Check sheet for the modelled part. Datum: model origin and axes. Units: mm. A direction names the side the tool comes from. Coordinates: 2 decimals unless noted, no trailing zeros. Write each loop counter-clockwise with the first axis right and the second up, starting at its lowest first coordinate (ties: lowest second). Pieces come first, ordered by that corner, then holes. Notation, with made-up numbers: (32, -38.5) - (42, -38.5) arc R30 cw to (42, -16.5) - close; hole circle Ø4 at (67, 66.25). An arc over 180 degrees is marked (long way). Write each question's results on one line, items separated by ' | '.
from build123d import *

# Parameters (mm, degrees)
F0_W     = 30.48
F0_H     = 25.4
F0_W_2   = 25.4
F0_H_2   = 20.32
F1_DEPTH = 44.45
F2_W     = 25.4
F2_H     = 20.32
F2_W_2   = 20.32
F2_H_2   = 15.24
F2_R     = 2.159
F3_DEPTH = 25.4
F4_R     = 2.159
F5_DEPTH = 5.08
F6_R     = 3.429
F6_W     = 8.128
F6_H     = 3.048
F7_DEPTH = 25.4
F8_W     = 54.200325
F8_H     = 68.948708
F9_DEPTH = 12.7


with BuildPart() as f1:
    # F0 (on Top) → F1 (new body, symmetric)
    with BuildSketch(Plane.XY):
        Rectangle(F0_W, F0_H)
        Rectangle(F0_W_2, F0_H_2, mode=Mode.SUBTRACT)
    extrude(amount=F1_DEPTH, both=True)

    # F2 (on face) → F3 (join)
    with BuildSketch(Plane.XY.offset(44.45)):
        Rectangle(F2_W, F2_H)
        Rectangle(F2_W_2, F2_H_2, mode=Mode.SUBTRACT)
        Rectangle(F2_W_2, F2_H_2)
        with Locations((-6.35, 0)):
            Circle(F2_R, mode=Mode.SUBTRACT)
        with Locations((6.35, 0)):
            Circle(F2_R, mode=Mode.SUBTRACT)
    extrude(amount=-F3_DEPTH)

    # F4 (on face) → F5 (cut)
    with BuildSketch(Plane(origin=(0, 0, 19.05), x_dir=(1, 0, 0), z_dir=(0, 0, -1))):
        with Locations((6.35, 0)):
            Circle(F4_R)
        with Locations((-6.35, 0)):
            Circle(F4_R)
    extrude(amount=-F5_DEPTH, mode=Mode.SUBTRACT)

    # F6 (on face) → F7 (cut)
    with BuildSketch(Plane.XZ.offset(12.7)):
        with Locations((0, 8.001)):
            Circle(F6_R)
        with Locations((0, -8.4074)):
            Rectangle(F6_W, F6_H)
        with BuildLine():
            Line((-3.2258, -29.3624), (-3.2258, -32.1564))
            Line((-3.2258, -32.1564), (3.2258, -32.1564))
            Line((3.2258, -32.1564), (3.2258, -29.3624))
            ThreePointArc((3.2258, -29.3624), (0, -26.1366), (-3.2258, -29.3624))
        make_face()
    extrude(amount=-F7_DEPTH, mode=Mode.SUBTRACT)

    # F8 (on Front) → F9 (cut, symmetric)
    with BuildSketch(Plane.XZ):
        with Locations((2.120081, 16.499758)):
            Rectangle(F8_W, F8_H)
    extrude(amount=F9_DEPTH, both=True, mode=Mode.SUBTRACT)


solid = f1.part
1. Sectioned sample at D-D (z = -19.5). Record the cut outline in (x, y).
Values follow:
outline: (-15.24, -12.7) - (15.24, -12.7) - (15.24, 12.7) - (-15.24, 12.7) - close; hole (-12.7, -10.16) - (12.7, -10.16) - (12.7, 10.16) - (-12.7, 10.16) - close
2. Material ranges on L1, parallel to X at y = -8.5, z = -26.75; L2, parallel to Y at x = -3, z = -27.5; L3, parallel to X at y = 11, z = -30.5, recorded low to high. Write a range as [from, to].
Values follow:
L1: x = [-15.24, -12.7], [12.7, 15.24] | L2: y = [-12.7, -10.16], [10.16, 12.7] | L3: x = [-15.24, -3.23], [3.23, 15.24]
3. Go/stop test with a flat-tipped pin: pin 1 (1 mm diameter, centred on x = 6.5, y = 8, fed in from +Z). Record where the tip stops, or that it passes through.
Values follow:
pin 1: passes through
4. Draft check along Y on faces 4 (the flat face through (0, -10.16, -34)), 5 (the flat face through (0, 11, -17.975)), 6 (the flat face through (0, 12.7, -34)). Enter one of: pulls with the +Y half, pulls with the -Y half, needs draft (parallel to the pull), parting line crosses it, or undercut.
Values follow:
face 4: undercut | face 5: needs draft | face 6: pulls with the +Y half
5. Access from +Z, -Z, +X, -X, +Y, -Y to the whole of each face (thin tool, end or side, straight path). Record for faces 1 (the flat face through (-15.24, 0, -31)), 2 (the flat face through (-12.7, 0, -31)), 3 (the flat face through (3.226, -11, -31)).
Values follow:
face 1: +Z, -Z, -X, +Y, -Y | face 2: +Z, -Z | face 3: +Y, -Y
6. Sectioned sample at B-B (x = -5.5). Record the cut outline in (y, z).
Values follow:
outline: (-12.7, -44.45) - (-10.16, -44.45) - (-10.16, -17.97) - (-12.7, -17.97) - close; (10.16, -44.45) - (12.7, -44.45) - (12.7, -17.97) - (10.16, -17.97) - close
7. Sectioned sample at C-C (x = 0). Record the cut outline in (y, z).
Values follow:
outline: (-12.7, -44.45) - (-10.16, -44.45) - (-10.16, -32.16) - (-12.7, -32.16) - close; (-12.7, -26.14) - (-10.16, -26.14) - (-10.16, -17.97) - (-12.7, -17.97) - close; (10.16, -44.45) - (12.7, -44.45) - (12.7, -32.16) - (10.16, -32.16) - close; (10.16, -26.14) - (12.7, -26.14) - (12.7, -17.97) - (10.16, -17.97) - close
8. Sectioned sample at A-A (y = 2.25). Record the cut outline in (x, z).
Values follow:
outline: (-15.24, -44.45) - (-12.7, -44.45) - (-12.7, -17.97) - (-15.24, -17.97) - close; (12.7, -44.45) - (15.24, -44.45) - (15.24, -17.97) - (12.7, -17.97) - close
